```python
from build123d import *

# Parameters (mm, degrees)
SKETCH1_W           = 101.6
SKETCH1_H           = 50.8
BOSS_EXTRUDE1_DEPTH = 50.8
SKETCH2_R           = 7.9375
CUT_EXTRUDE1_DEPTH  = 6.35
SKETCH3_R           = 6.35
CUT_EXTRUDE2_DEPTH  = 102.6
SKETCH4_R           = 5.3975
CUT_EXTRUDE3_DEPTH  = 34.29
SHELL9_T            = -2.54
SKETCH5_R           = 7.022033088
CUT_EXTRUDE4_DEPTH  = 96.52
SKETCH7_R           = 7.9375
BOSS_EXTRUDE3_DEPTH = 11.43
SKETCH9_R           = 5.08
CUT_EXTRUDE5_DEPTH  = 34.29
SKETCH10_R          = 6.35
BOSS_EXTRUDE4_DEPTH = 2.54


with BuildPart() as part:
    # Sketch1 → Boss-Extrude1 (new body)
    with BuildSketch(Plane.XY):
        Rectangle(SKETCH1_W, SKETCH1_H)
    extrude(amount=-BOSS_EXTRUDE1_DEPTH)

    # Sketch2 → Cut-Extrude1 (cut)
    with BuildSketch(Plane(origin=(50.8, 0, 0), x_dir=(0, 0, -1), z_dir=(1, 0, 0))):
        with Locations((25.4, 1.27)):
            Circle(SKETCH2_R)
    extrude(amount=-CUT_EXTRUDE1_DEPTH, mode=Mode.SUBTRACT)

    # Sketch3 → Cut-Extrude2 (cut, through all)
    with BuildSketch(Plane(origin=(50.8, 0, 0), x_dir=(0, 0, -1), z_dir=(1, 0, 0))):
        with Locations((25.4, 1.27)):
            Circle(SKETCH3_R)
    extrude(amount=-CUT_EXTRUDE2_DEPTH, mode=Mode.SUBTRACT)

    # Sketch4 → Cut-Extrude3 (cut)
    with BuildSketch(Plane(origin=(0, 0, -50.8), x_dir=(-1, 0, 0), z_dir=(0, 0, -1))):
        with Locations((0, 11.461907579)):
            Circle(SKETCH4_R)
    extrude(amount=-CUT_EXTRUDE3_DEPTH, mode=Mode.SUBTRACT)

    # Shell9
    shell9_openings = [part.faces().sort_by_distance(p)[0] for p in [
        (0, 25.4, -25.4),
    ]]
    offset(amount=SHELL9_T, openings=shell9_openings, kind=Kind.INTERSECTION)

    # Sketch5 → Cut-Extrude4 (cut)
    with BuildSketch(Plane.ZY.offset(-48.26)):
        with Locations((-25.037035013, 8.282646085)):
            Circle(SKETCH5_R)
    extrude(amount=CUT_EXTRUDE4_DEPTH, mode=Mode.SUBTRACT)

    # Sketch7 → Boss-Extrude3 (add)
    with BuildSketch(Plane.XY.offset(-13.97)):
        with Locations((0, 11.461907579)):
            Circle(SKETCH7_R)
    extrude(amount=BOSS_EXTRUDE3_DEPTH)

    # Sketch9 → Cut-Extrude5 (cut)
    with BuildSketch(Plane.XY):
        with Locations((0, 11.461907579)):
            Circle(SKETCH9_R)
    extrude(amount=-CUT_EXTRUDE5_DEPTH, mode=Mode.SUBTRACT)

    # Sketch10 → Boss-Extrude4 (add)
    with BuildSketch(Plane.ZY.offset(50.8)):
        with Locations((-25.4, 1.27)):
            Circle(SKETCH10_R)
    extrude(amount=-BOSS_EXTRUDE4_DEPTH)


solid = part.part
```
Work out the finished part from the listing and answer in its coordinate system (mm). A direction names the side the tool comes from. Coordinates: 2 decimals unless noted, no trailing zeros. Write each loop counter-clockwise with the first axis right and the second up, starting at its lowest first coordinate (ties: lowest second). Pieces come first, ordered by that corner, then holes. Notation, with made-up numbers: (12, -29) - (17, -29) arc R22 ccw to (17, 10) - close; hole circle Ø1 at (50.5, 86). An arc over 180 degrees is marked (long way). Answer as a JSON object with one key per item and string values.
Q1. Which of the six approach directions +Z, -Z, +X, -X, +Y, -Y give full straight-line access (tool end or side, diameter ignored) to faces 5 (the flat face through (-1, -25.4, -25)), 6 (the cylindrical face through (-1.26, -5.08, -25.55)), 7 (the cylindrical face through (-2.54, -7.62, -25.58))?
Results list:
{"face 5": "+Z, -Z, +X, -X, -Y", "face 6": "+X", "face 7": "none"}
Q2. Find section C-C (x = 0). Write down the section's boundary in (y, z).
Results list:
{"outline": "(-25.4, -50.8) - (6.06, -50.8) - (6.06, -31.7) arc R7.02 cw to (4.43, -30.91) arc R6.35 cw (long way) to (3.84, -19.6) arc R7.02 cw to (6.06, -18.37) - (6.06, -16.51) - (6.38, -16.51) - (6.38, 0) - (-25.4, 0) - close; (16.54, -16.51) - (16.86, -16.51) - (16.86, -50.8) - (25.4, -50.8) - (25.4, -48.26) - (19.4, -48.26) - (19.4, -2.54) - (25.4, -2.54) - (25.4, 0) - (16.54, 0) - close; hole (-22.86, -48.26) - (3.52, -48.26) - (3.52, -34) arc R8.89 cw (long way) to (3.52, -16.8) - (3.52, -2.54) - (-22.86, -2.54) - close"}
Q3. Find section D-D (z = -25.4). State how many separate pieces and enclosed holes the cut face has, plus the area to 3 significant figures.
Results list:
{"separate pieces": "3", "enclosed holes": "1", "area": "744 mm^2"}
Q4. Find section B-B (y = 1.27). Write down the section's boundary in (x, z).
Results list:
{"outline": "(-50.8, -50.8) - (50.8, -50.8) - (50.8, -33.34) - (44.45, -33.34) - (44.45, -31.75) - (-48.26, -31.75) - (-48.26, -19.05) - (44.45, -19.05) - (44.45, -17.46) - (50.8, -17.46) - (50.8, 0) - (-50.8, 0) - close; hole (-48.26, -48.26) - (48.26, -48.26) - (48.26, -35.88) - (41.91, -35.88) - (41.91, -34.29) - (-48.26, -34.29) - close; hole (-48.26, -16.51) - (41.91, -16.51) - (41.91, -14.92) - (48.26, -14.92) - (48.26, -2.54) - (-48.26, -2.54) - close"}
Q5. Given pin 1 Ø1.5 at (x, z) = (-8, -16.5) entering from +Y; pin 2 Ø1.5 at (x, z) = (14, -10) entering from +Y; pin 3 Ø1 at (x, z) = (-20.5, -34) entering from +Y, each flat-ended and moving along its own axis, determine where each tip first touches the part or whether it passes through.
Results list:
{"pin 1": "stops at y = 14.69", "pin 2": "stops at y = -22.86", "pin 3": "stops at y = 4.93"}
Q6. Find section A-A (z = -39). Write down the section's boundary in (x, y) (1 decimal).
Results list:
{"outline": "(-50.8, -25.4) - (50.8, -25.4) - (50.8, 25.4) - (48.3, 25.4) - (48.3, -22.9) - (-48.3, -22.9) - (-48.3, 25.4) - (-50.8, 25.4) - close; circle Ø15.9 at (0, 11.5); hole circle Ø10.8 at (0, 11.5)"}
Q7. For a pull along Y with two mould halves and no side action, classify faces 1 (the flat face through (-50.8, 0, -26)), 2 (the cylindrical face through (0.703, 16.813, -37.705)), 3 (the flat face through (-4, 25.4, -50)), 4 (the cylindrical face through (47.67, -6.48, -23.68)) as pulls with the +Y half, pulls with the -Y half, needs draft (parallel to the pull), parting line crosses it, or undercut.
Results list:
{"face 1": "needs draft", "face 2": "undercut", "face 3": "pulls with the +Y half", "face 4": "undercut"}
Q8. Consider L1, parallel to Z at x = 48, y = 1; L2, parallel to Y at x = 0, z = -9; L3, parallel to Z at x = 21, y = 1.27. Determine where each line is inside the solid, lowest interval first. Write a range as from..to.
Results list:
{"L1": "z = -50.8..-48.26, -35.87..-33.33, -17.47..-14.93, -2.54..0", "L2": "y = -25.4..-22.86, 3.52..6.38, 16.54..19.4", "L3": "z = -50.8..-48.26, -34.29..-31.75, -19.05..-16.51, -2.54..0"}
